Autodesk Inventor part; units mm, degrees
ref_plane "YZ Plane" through (0, 0, 0) normal (1, 0, 0) x (0, 1, 0)
ref_plane "XY Plane" through (0, 0, 0) normal (0, 0, 1) x (1, 0, 0)
ref_plane "Work Plane1" through (0, 0, 6.35) normal (0, 0, -1) x (-1, 0, 0)
sketch "Sketch1" plane through (0, 0, 0) normal (0, 0, 1) x (1, 0, 0)
  line L0 (0, -6.0638) -> (7.1374, -6.0638)
  line L1 (7.1374, -6.0638) -> (7.1374, -19.05)
  line L2 (7.1374, -19.05) -> (11.1772, -19.05)
  line L3 (11.1772, -19.05) -> (11.1772, 0)
  line L4 (11.1772, 0) -> (15.367, 0)
  line L5 (15.367, 0) -> (15.367, 4.8514)
  line L6 (15.367, 4.8514) -> (12.7524, 23.4552)
  arc A0 (12.7524, 23.4552) -> (1.5875, 25.4) centre (1.5875, -7.62) ccw
  line L7 (-21.5138, 0) -> (21.5138, 0) construction
  line L8 (0, -28.0365) -> (0, 34.8691) construction
  line L9 (0, -6.0638) -> (-7.1374, -6.0638)
  line L10 (-7.1374, -6.0638) -> (-7.1374, -19.05)
  line L11 (-7.1374, -19.05) -> (-11.1772, -19.05)
  line L12 (-11.1772, -19.05) -> (-11.1772, 0)
  line L13 (-11.1772, 0) -> (-15.367, 0)
  line L14 (-15.367, 0) -> (-15.367, 4.8514)
  line L15 (-15.367, 4.8514) -> (-12.7524, 23.4552)
  line L16 (7.1374, -12.7) -> (11.1772, -12.7) construction
  line L17 (-7.1374, -12.7) -> (-11.1772, -12.7) construction
  line L18 (1.5875, 25.4) -> (0, 25.4)
  arc A1 (-1.5875, 25.4) -> (-12.7524, 23.4552) centre (-1.5875, -7.62) ccw
  line L19 (-1.5875, 25.4) -> (0, 25.4)
  point P0 (0, 0)
  dimension "d1" = 30.734
  dimension "d2" = 4.1898
  dimension "d3" = 4.0398
  dimension "d4" = 6.35
  dimension "d5" = 12.7
  dimension "d6" = 17.5514
  dimension "d7" = 8
  dimension "d8" = 1.5875
  dimension "d9" = 38.1
  dimension "d10" = 33.02
extrude "Extrusion1" add sketch "Sketch1" along normal blind 12.7
hole "Hole1" at (11.1772, -12.7, 6.35) direction (-1, 0, 0) diameter 4.8006 end through all
fillet "Fillet1" radius 6.35 4 edges at (9.1573, -19.05, 12.7) (9.1573, -19.05, 0) (-9.1573, -19.05, 12.7) (-9.1573, -19.05, 0)
sketch "Sketch2" plane through (11.1772, 0, 12.7) normal (1, 0, 0) x (0, 0, -1)
  line L0 (12.7, 0) -> (0, 0)
  line L1 (0, -12.7) -> (0, 0) construction
  line L2 (12.7, -12.7) -> (12.7, 0) construction
  line L3 (0, -3.361) -> (12.7, -7.9834)
  line L4 (12.7, 0) -> (12.7, -7.9834)
  line L5 (0, -3.361) -> (0, 0)
  point P0 (6.35, -12.7)
  dimension "d23" = 6.604
  dimension "d24" = 20
extrude "Extrusion2" add sketch "Sketch2" along normal up to surface (4.1898 mm away)
mirror "Mirror1" about plane through (0, 0, 0) normal (1, 0, 0) of "Extrusion2"
ref_plane "Work Plane1" through (0, 0, 6.35) normal (0, 0, -1) x (-1, 0, 0)
ref_plane "Work Plane2" through (11.1772, -12.7, 0) normal (0, 1, 0) x (-1, 0, 0)
equation "\"d1\" = finger_w"
equation "\"d2\" = finger_link_w + tol"
equation "\"d3\" = finger_link_w - tol"
equation "\"d4\" = 0.5 * finger_t"
equation "\"d11\" = finger_t"
equation "\"d15\" = bore_clearance"
equation "\"d22\" = 0.5 * finger_t"
equation "\"d25\" = finger_t"
equation "\"finger_A_l\" = 57.15"
equation "\"finger_w\" = 30.734"
equation "\"finger_B_l\" = 38.1"
equation "\"finger_link_w\" = 4.1148"
equation "\"tolerance1\" = 0.15"
equation "\"tol\" = 0.5 * tolerance1"
equation "\"finger_t\" = 12.7"
equation "\"bore_press\" = 4.8006"
equation "\"bore_clearance\" = bore_press"
properties part number "finger_tip"
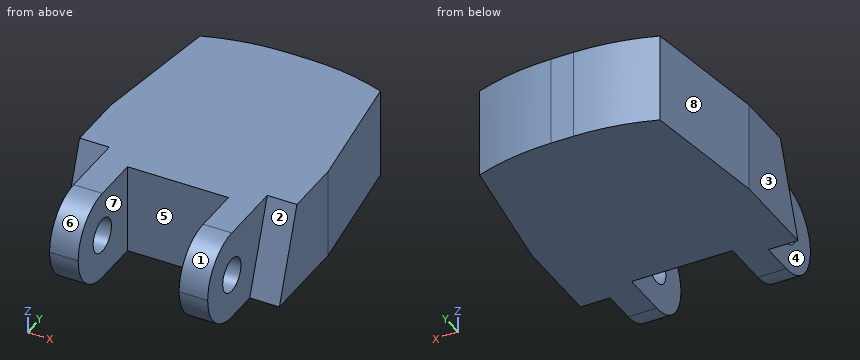
Geometry check sheet. Reference: the model listing, model coordinates, mm. Face numbers are marked on the shaded views. A direction names the side the tool comes from. Round coordinates to 2 decimals unless told otherwise and drop trailing zeros. Order: outer loops, then holes, each group sorted by start corner. A loop starts at its lowest first (then second) coordinate and runs counter-clockwise, first axis right, second up. Notation, with made-up numbers: (-38, 52.5) -> (-25, 52.5) arc R28 cw to (-25, 76.5) -> close; hole circle Ø2 at (83, 18.5). An arc over 180 degrees is marked (long way). Use one line per item in the form item = value.
1. Set-up check for the marked faces 1, 2, 3, 4 and 5: record each of +Z, -Z, +X, -X, +Y, -Y from which the full face is reachable in a straight line by a thin tool's end or side.
Working result:
face_1 = +Z, +X, -X, -Y
face_2 = +Z, +X, -Y
face_3 = +Z, -Z, -X, +Y, -Y
face_4 = +Z, -X, -Y
face_5 = +Z, -Z, -Y
2. Scan lines: line 1 along X through (y, z) = (-9.5, 2); line 2 along Z through (x, y) = (-8.55, -12.7); line 3 along Y through (x, z) = (-9, 6.35). Record each from-to range of solid material in increasing order. Write a range as from..to.
Working result:
line_1 = -11.18..-7.14, 7.14..11.18
line_2 = 0..3.95, 8.75..12.7
line_3 = -19.05..-15.1, -10.3..24.56
3. Cross-section at B-B, the plane y = -12. Enter the section's corners in (x, z), plus the area to 3 significant figures.
Working result:
outline = (-11.18, 0) -> (-7.14, 0) -> (-7.14, 4.05) -> (-11.18, 4.05) -> close; (-11.18, 8.65) -> (-7.14, 8.65) -> (-7.14, 12.7) -> (-11.18, 12.7) -> close; (7.14, 0) -> (11.18, 0) -> (11.18, 4.05) -> (7.14, 4.05) -> close; (7.14, 8.65) -> (11.18, 8.65) -> (11.18, 12.7) -> (7.14, 12.7) -> close
area = 65.5 mm^2
4. Go/stop test with flat-tipped pins: pin 1 (5.5 mm diameter, centred on y = -12.7, z = 6.35, fed in from -X); pin 2 (1.5 mm diameter, centred on x = 7.5, z = 6, fed in from -Y); pin 3 (6 mm diameter, centred on y = -12.7, z = 6.35, fed in from +X); pin 4 (1 mm diameter, centred on x = 12, z = 10.5, fed in from +Y). Record where each tip stops, or that it passes through.
Working result:
pin_1 = -11.18
pin_2 = -19.05
pin_3 = 11.18
pin_4 = 23.88
5. Mould release check, pull along X, two halves, no side actions. Record for the marked faces 6, 7 and 8: pulls with the +X half, pulls with the -X half, needs draft (parallel to the pull), parting line crosses it, or undercut.
Working result:
face_6 = needs draft
face_7 = undercut
face_8 = pulls with the -X half
6. Cross-section at C-C, the plane z = 9.25. Enter the section's corners in (x, y).
Working result:
outline = (-15.37, -4.62) -> (-11.18, -4.62) -> (-11.18, -18.35) -> (-7.14, -18.35) -> (-7.14, -6.06) -> (7.14, -6.06) -> (7.14, -18.35) -> (11.18, -18.35) -> (11.18, -4.62) -> (15.37, -4.62) -> (15.37, 4.85) -> (12.75, 23.46) arc R33.02 ccw to (1.59, 25.4) -> (-1.59, 25.4) arc R33.02 ccw to (-12.75, 23.46) -> (-15.37, 4.85) -> close
7. Cross-section at A-A, the plane z = 7.25. Enter the section's corners in (x, y).
Working result:
outline = (-15.37, -5.34) -> (-11.18, -5.34) -> (-11.18, -10.47) -> (-7.14, -10.47) -> (-7.14, -6.06) -> (7.14, -6.06) -> (7.14, -10.47) -> (11.18, -10.47) -> (11.18, -5.34) -> (15.37, -5.34) -> (15.37, 4.85) -> (12.75, 23.46) arc R33.02 ccw to (1.59, 25.4) -> (-1.59, 25.4) arc R33.02 ccw to (-12.75, 23.46) -> (-15.37, 4.85) -> close; (-11.18, -18.99) -> (-7.14, -18.99) -> (-7.14, -14.93) -> (-11.18, -14.93) -> close; (7.14, -18.99) -> (11.18, -18.99) -> (11.18, -14.93) -> (7.14, -14.93) -> close
